Autodesk Inventor part; units mm, degrees
ref_plane "YZ Plane" through (0, 0, 0) normal (1, 0, 0) x (0, 1, 0)
ref_plane "XZ Plane" through (0, 0, 0) normal (0, 1, 0) x (-1, 0, 0)
ref_plane "XY Plane" through (0, 0, 0) normal (0, 0, 1) x (1, 0, 0)
sketch "Sketch1" plane through (0, 0, 0) normal (0, 0, 1) x (1, 0, 0)
  circle A0 centre (0, 0) radius 361.95
  circle A1 centre (0, 0) radius 393.7
  dimension "d0" = 723.9
  dimension "d1" = 787.4
extrude "Extrusion1" add sketch "Sketch1" along normal blind 304.8
sketch "Sketch2" plane through (0, 0, 304.8) normal (0, 0, 1) x (1, 0, 0)
  circle A0 centre (0, 0) radius 393.7
  circle A1 centre (0, 0) radius 396.621
  circle A2 centre (0, 0) radius 399.796
  dimension "d4" = 793.242
  dimension "d5" = 799.592
extrude "Extrusion2" add sketch "Sketch2" against normal blind 50.8 contours A1
extrude "Extrusion3" add sketch "Sketch2" against normal blind 25.4 contours A2
chamfer "Chamfer1" distance 2.921 angle 45 1 edges at (-393.7, 0, 254)
sketch "Sketch3" plane through (0, 0, 0) normal (0, 0, -1) x (-1, 0, 0)
  circle A0 centre (0, 0) radius 380.746
  circle A1 centre (0, 0) radius 361.95
  dimension "d13" = 761.492
extrude "Extrusion4" add sketch "Sketch3" along normal blind 12.7
fillet "Fillet1" radius 0.7937 2 edges at (380.746, 0, 0) (-396.621, 0, 279.4)
chamfer "Chamfer2" distance 0.7937 angle 45 1 edges at (380.746, 0, -12.7)
chamfer "Chamfer3" distance 0.7937 angle 45 1 edges at (-399.796, 0, 279.4)
sketch "Sketch4" plane through (0, 0, 0) normal (1, 0, 0) x (0, 1, 0)
  line L0 (396.621, 278.6062) -> (396.621, 254) construction
  line L1 (-399.796, 304.8) -> (399.796, 304.8) construction
  line L2 (396.621, 273.05) -> (394.8409, 271.2699)
  arc A0 (394.8409, 271.2699) -> (393.446, 267.9023) centre (398.2085, 267.9023) ccw
  line L3 (393.446, 267.9023) -> (393.446, 267.0852)
  arc A1 (393.446, 267.0852) -> (394.8409, 263.7176) centre (398.2085, 267.0852) ccw
  line L4 (394.8409, 263.7176) -> (396.621, 261.9375)
  line L5 (396.621, 261.9375) -> (396.621, 273.05)
  line L6 (0, -60.96) -> (0, 365.76)
  point P0 (0, 0)
  dimension "d23" = 11.1125
  dimension "d24" = 3.175
  dimension "d25" = 4.7625
  dimension "d26" = 31.75
  dimension "d27" = 45
revolve "Revolution1" cut sketch "Sketch4" angle 360 about axis through (0, 0, -10) along (0, 0, 1)
equation "\"d10\" = -0.5 * d1 + 0.5 * d4"
properties part number "A1-19037-200-06 HCWI liner - pup" material "Iron, HCWI"
CAD build for the part. Positions are in the model's coordinates, mm. A direction names the side the tool comes from. Give positions to 0.01 mm unless a question says otherwise; leave off trailing zeros. Order: outer loops, then holes, each group sorted by start corner. A loop starts at its lowest first (then second) coordinate and runs counter-clockwise, first axis right, second up. Notation, with made-up numbers: (-36, 51.25) - (-15, 51.25) arc R24 cw to (-15, 86.25) - close; hole circle Ø10 at (-24, 33). An arc over 180 degrees is marked (long way). Answer in a Markdown table with one row per item.
1. Tool access for faces 1 (the conical face through (385.56, -85.62, 271.38)), 2 (the cylindrical face through (381.334, 120.088, 292.669)), 3 (the flat face through (-206, 323, 0)): list every direction of +Z, -Z, +X, -X, +Y, -Y with a clear straight run to the whole face (end or side of a thin tool).
Data:
| item | result |
|---|---|
| face 1 | none |
| face 2 | +Z, -Z |
| face 3 | -Z |
2. Pull direction Z, two halves, no side cores. Call faces 4 (the cylindrical face through (-384.09, -85.29, 267.49)), 5 (the cylindrical face through (375.52, -118.26, 123.78)), 6 (the flat face through (-61, 357, 304.8)): pulls with the +Z half, pulls with the -Z half, needs draft (parallel to the pull), parting line crosses it, or undercut.
Data:
| item | result |
|---|---|
| face 4 | undercut |
| face 5 | needs draft |
| face 6 | pulls with the +Z half |
3. Flat gauge pins, fed straight in: pin 1 (10 mm diameter, centred on x = -90, z = 129.5, fed in from -Y); pin 2 (12 mm diameter, centred on y = 263.5, z = 131.5, fed in from +X); pin 3 (4 mm diameter, centred on x = 59, z = 228, fed in from -Y). Where does each tip first touch, or does it go through?
Data:
| item | result |
|---|---|
| pin 1 | stops at y = -384.41 |
| pin 2 | stops at x = 297.81 |
| pin 3 | stops at y = -389.55 |
4. Saw through at A-A, the plane z = 100.5. Give the cut face in (x, y), plus the area to 3 significant figures.
Data:
| item | result |
|---|---|
| outline | circle Ø787.4 at (0, 0); hole circle Ø723.9 at (0, 0) |
| area | 75,400 mm² |
5. Probe probe 1 along Y at (x, z) = (0, 194.5); probe 2 along Y at (x, z) = (0, -9); probe 3 along X at (y, z) = (211.5, 104.5). List the from-to ranges inside material, lowest first. Write a range as [from, to].
Data:
| item | result |
|---|---|
| probe 1 | y = [-393.7, -361.95], [361.95, 393.7] |
| probe 2 | y = [-380.75, -361.95], [361.95, 380.75] |
| probe 3 | x = [-332.07, -293.73], [293.73, 332.07] |
